from build123d import *

# Parameters (mm, degrees)
F1_DEPTH = 304.8
F2_T     = -2.3622
F4_DEPTH = 203.2
F6_DEPTH = 76.498957
F8_DEPTH = 76.498957


with BuildPart() as f1:
    # F0 (on Top) → F1 (new body)
    with BuildSketch(Plane.XY):
        with BuildLine():
            Line((-31.898979, -38.248979), (31.898979, -38.248979))
            ThreePointArc((31.898979, -38.248979), (36.389107, -36.389107), (38.248979, -31.898979))
            Line((38.248979, -31.898979), (38.248979, 31.898979))
            ThreePointArc((38.248979, 31.898979), (36.389107, 36.389107), (31.898979, 38.248979))
            Line((31.898979, 38.248979), (-31.898979, 38.248979))
            ThreePointArc((-31.898979, 38.248979), (-36.389107, 36.389107), (-38.248979, 31.898979))
            Line((-38.248979, 31.898979), (-38.248979, -31.898979))
            ThreePointArc((-38.248979, -31.898979), (-36.389107, -36.389107), (-31.898979, -38.248979))
        make_face()
    extrude(amount=F1_DEPTH)

    # F2
    f2_openings = [f1.faces().sort_by_distance(p)[0] for p in [
        (0, 0, 304.8),
        (0, 0, 0),
    ]]
    offset(amount=F2_T, openings=f2_openings)

    # F3 (on face) → F4 (cut)
    with BuildSketch(Plane.XY.offset(304.8)):
        Polygon((-35.886779, -31.898979), (-38.248979, -31.898979), (-38.248979, -60.503662), (63.648979, -60.503662), (63.648979, 38.248979), (31.898979, 38.248979), (31.898979, 35.886779), align=None)
    extrude(amount=-F4_DEPTH, mode=Mode.SUBTRACT)

    # F5 (on face) → F6 (cut, through all)
    with BuildSketch(Plane(origin=(-38.248979, 0, 0), x_dir=(0, -1, 0), z_dir=(-1, 0, 0))):
        with BuildLine():
            ThreePointArc((-3.5, 248.3), (0, 244.8), (3.5, 248.3))
            Line((3.5, 248.3), (3.5, 291.3))
            ThreePointArc((3.5, 291.3), (0, 294.8), (-3.5, 291.3))
            Line((-3.5, 291.3), (-3.5, 248.3))
        make_face()
        with BuildLine():
            ThreePointArc((-3.5, 108.299998), (2e-06, 104.799998), (3.5, 108.300002))
            Line((3.5, 108.300002), (3.5, 151.300002))
            ThreePointArc((3.5, 151.300002), (-2e-06, 154.799998), (-3.5, 151.299998))
            Line((-3.5, 151.299998), (-3.5, 108.299998))
        make_face()
    extrude(amount=-F6_DEPTH, mode=Mode.SUBTRACT)

    # F7 (on face) → F8 (cut, through all)
    with BuildSketch(Plane(origin=(0, 38.248979, 0), x_dir=(-1, 0, 0), z_dir=(0, 1, 0))):
        with BuildLine():
            ThreePointArc((-3.5, 248.300001), (0, 244.800001), (3.5, 248.300001))
            Line((3.5, 248.300001), (3.5, 291.299999))
            ThreePointArc((3.5, 291.299999), (0, 294.800001), (-3.5, 291.299999))
            Line((-3.5, 291.299999), (-3.5, 248.300001))
        make_face()
        with BuildLine():
            ThreePointArc((-3.5, 108.300001), (0, 104.800001), (3.5, 108.300001))
            Line((3.5, 108.300001), (3.5, 151.299999))
            ThreePointArc((3.5, 151.299999), (0, 154.799999), (-3.5, 151.299999))
            Line((-3.5, 151.299999), (-3.5, 108.300001))
        make_face()
    extrude(amount=-F8_DEPTH, mode=Mode.SUBTRACT)


solid = f1.part
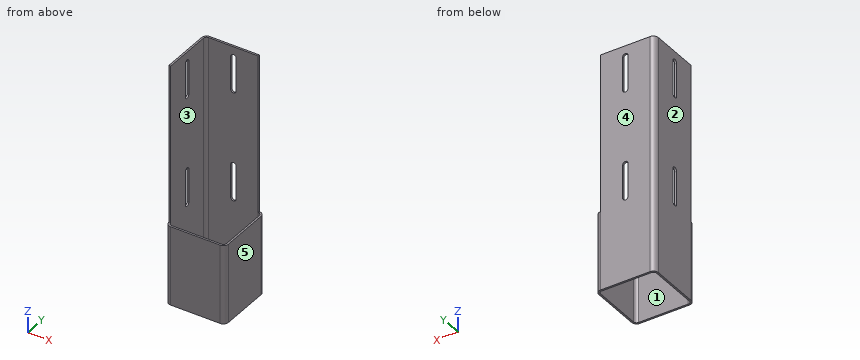
Design review of the part built by this model. Coordinates are the model's own, in mm. Face numbers are marked on the shaded views. A direction names the side the tool comes from. Coordinates: 2 decimals unless noted, no trailing zeros. Write each loop counter-clockwise with the first axis right and the second up, starting at its lowest first coordinate (ties: lowest second). Pieces come first, ordered by that corner, then holes. Notation, with made-up numbers: (14.5, 9.5) - (28.5, 9.5) arc R20 ccw to (28.5, 33.5) - close; hole circle Ø8 at (75.5, -18). An arc over 180 degrees is marked (long way). Use one line per item in the form item = value.
Q1. For probe 1 along Y at (x, z) = (5, 14.5); probe 2 along Y at (x, z) = (29, 213), list the stretches that pass through material, from the lowest coordinate up.
Taken from the geometry:
probe_1 = -38.25 to -35.89, 35.89 to 38.25
probe_2 = 35.89 to 38.25
Q2. Consider section D-D (y = 0). Write out the cut boundary in (x, z).
Taken from the geometry:
outline = (-38.25, 0) - (-35.89, 0) - (-35.89, 104.8) - (-38.25, 104.8) - close; (-38.25, 154.8) - (-35.89, 154.8) - (-35.89, 244.8) - (-38.25, 244.8) - close; (-38.25, 294.8) - (-35.89, 294.8) - (-35.89, 304.8) - (-38.25, 304.8) - close; (35.89, 0) - (38.25, 0) - (38.25, 101.6) - (35.89, 101.6) - close
Q3. Insertion check: pin 1 Ø1.2 at (x, z) = (-37, 266.5) entering from +Y; pin 2 Ø2.5 at (y, z) = (36.5, 130) entering from +X; pin 3 Ø2.5 at (x, z) = (-37.5, 267.5) entering from -Y. Each pin has a flat end and moves straight along its axis. Give the tip position at first contact, or say it passes through.
Taken from the geometry:
pin_1 = 36.38
pin_2 = 31.9
pin_3 = -31.9
Q4. Machinability: for the marked faces 1 and 2, which of the approach directions +Z, -Z, +X, -X, +Y, -Y give a long, thin tool a straight path to every point of the face, cutting with its end or side? Answer none if there is none.
Taken from the geometry:
face_1 = +Z, -Z
face_2 = +Z, -Z, -X, +Y, -Y
Q5. Consider section A-A (x = 0). Write out the cut boundary in (y, z), plus the area to 3 significant figures.
Taken from the geometry:
outline = (-38.25, 0) - (-35.89, 0) - (-35.89, 101.6) - (-38.25, 101.6) - close; (35.89, 0) - (38.25, 0) - (38.25, 104.8) - (35.89, 104.8) - close; (35.89, 154.8) - (38.25, 154.8) - (38.25, 244.8) - (35.89, 244.8) - close; (35.89, 294.8) - (38.25, 294.8) - (38.25, 304.8) - (35.89, 304.8) - close
area = 724 mm^2
Q6. The part is to be moulded in two halves that separate along X. For the marked faces 3, 4 and 5, say which applies: +X half, -X half, draft (parallel to the pull), parting line (faces both ways), or undercut.
Taken from the geometry:
face_3 = undercut
face_4 = draft
face_5 = +X half
Q7. Consider section C-C (z = 268.5). Write out the cut boundary in (x, y).
Taken from the geometry:
outline = (-38.25, -31.9) - (-35.89, -31.9) - (-35.89, -3.5) - (-38.25, -3.5) - close; (-38.25, 3.5) - (-35.89, 3.5) - (-35.89, 31.9) arc R3.99 cw to (-31.9, 35.89) - (-3.5, 35.89) - (-3.5, 38.25) - (-31.9, 38.25) arc R6.35 ccw to (-38.25, 31.9) - close; (3.5, 35.89) - (31.9, 35.89) - (31.9, 38.25) - (3.5, 38.25) - close
Q8. Consider section B-B (y = 12.5). Write out the cut boundary in (x, z).
Taken from the geometry:
outline = (-38.25, 0) - (-35.89, 0) - (-35.89, 304.8) - (-38.25, 304.8) - close; (35.89, 0) - (38.25, 0) - (38.25, 101.6) - (35.89, 101.6) - close
